Here's the drawing with two shaded views (mm, measured from the low corner). I have some questions. A direction names the side the tool comes from. Round coordinates to 2 decimals unless told otherwise and drop trailing zeros. Loops run counter-clockwise (first coordinate to the right, second up) from the corner with the lowest first, then second, coordinate; pieces in that order, holes last. Notation, with made-up numbers: (13, 42) -> (41, 42) arc R6 cw to (41, 49) -> close; hole circle Ø7 at (89, 77). An arc over 180 degrees is marked (long way). Write item = value, one per line.
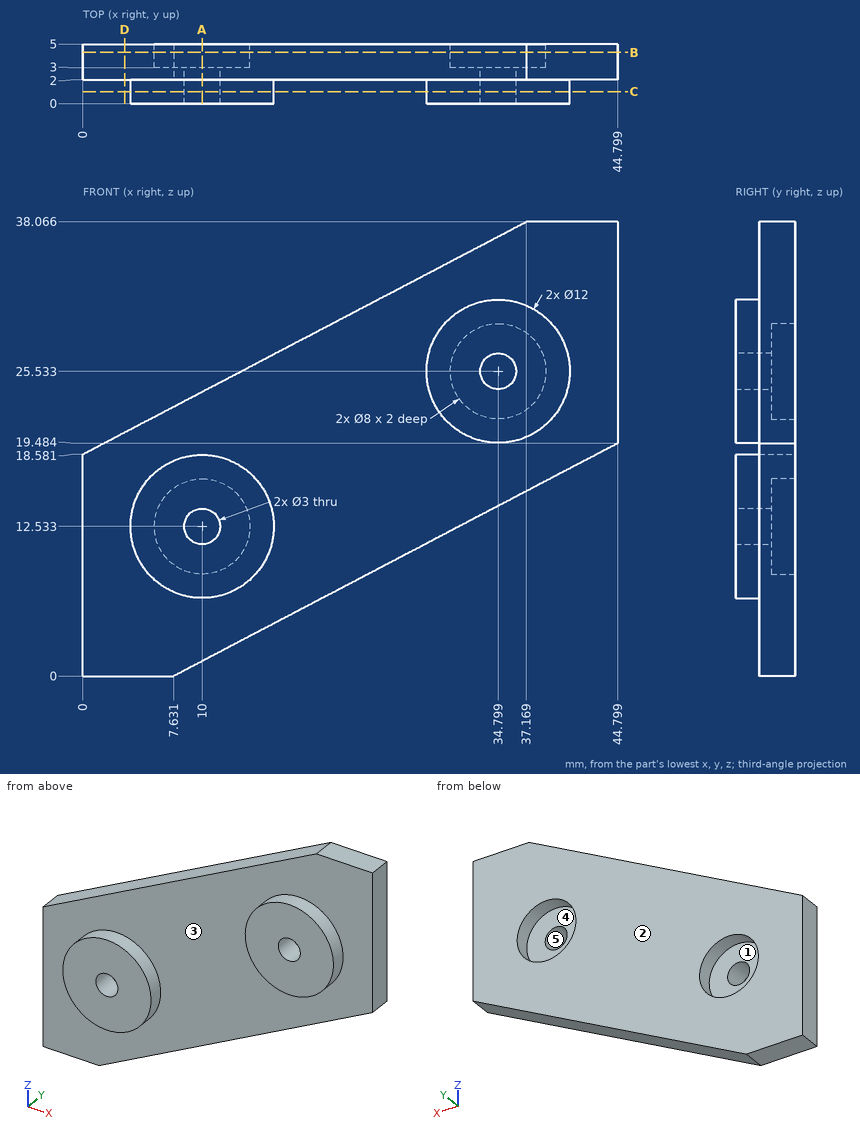
1. Suppose I cut it at D-D, the plane x = 3.5. List the corners of the cut face in (y, z) for me.
Entries:
outline = (2, 0) -> (5, 0) -> (5, 20.42) -> (2, 20.42) -> close
2. I need wall thicknesses on line 1 (Y direction, x = 24.5, z = 29); line 2 (Z direction, x = 8.5, y = 4.2) (1 decimal); line 3 (Z direction, x = 9.5, y = 0.75) (1 decimal). Which ranges of each line are inside material? Lowest first, please. Write a range as [from, to].
Entries:
line_1 = [2, 5]
line_2 = [0.5, 8.8], [16.2, 23]
line_3 = [6.6, 11.1], [13.9, 18.5]
3. We'd pull the mould along X, two halves only. Please class the marked faces 1 and 2: released by +X, released by -X, zero draft, split by the parting line, or undercut.
Entries:
face_1 = undercut
face_2 = zero draft
4. Suppose I cut it at B-B, the plane y = 4.3. List the corners of the cut face in (x, z) for me (1 decimal).
Entries:
outline = (0, 0) -> (7.6, 0) -> (44.8, 19.5) -> (44.8, 38.1) -> (37.2, 38.1) -> (0, 18.6) -> close; hole circle Ø8 at (10, 12.5); hole circle Ø8 at (34.8, 25.5)
5. Suppose I cut it at C-C, the plane y = 1. List the corners of the cut face in (x, z) for me.
Entries:
outline = circle Ø12 at (10, 12.53); circle Ø12 at (34.8, 25.53); hole circle Ø3 at (10, 12.53); hole circle Ø3 at (34.8, 25.53)
6. For the marked faces 3, 4 and 5, which set-ups out of +Z, -Z, +X, -X, +Y, -Y let a thin tool reach every point of the face, with its end or its side?
Entries:
face_3 = -Y
face_4 = +Y
face_5 = +Y, -Y
7. I'm going to push flat-ended pins straight in: pin 1 (2 mm diameter, centred on x = 26, y = 1.5, fed in from +Z) (1 decimal); pin 2 (2.5 mm diameter, centred on x = 36.5, z = 27, fed in from +Y); pin 3 (19 mm diameter, centred on x = 29.5, z = 23.5, fed in from -Y); pin 4 (2 mm diameter, centred on y = 4.5, z = 6.5, fed in from +X) (1 decimal). Where does each tip first touch, or does it pass through?
Entries:
pin_1 = 32.7
pin_2 = 3
pin_3 = 0
pin_4 = 21.9
8. Suppose I cut it at A-A, the plane x = 10. List the corners of the cut face in (y, z) for me.
Entries:
outline = (0, 6.53) -> (2, 6.53) -> (2, 1.24) -> (5, 1.24) -> (5, 8.53) -> (3, 8.53) -> (3, 11.03) -> (0, 11.03) -> close; (0, 14.03) -> (3, 14.03) -> (3, 16.53) -> (5, 16.53) -> (5, 23.82) -> (2, 23.82) -> (2, 18.53) -> (0, 18.53) -> close
